Geometry check sheet. Reference: the model listing, model coordinates, mm. A direction names the side the tool comes from. Coordinates: 2 decimals unless noted, no trailing zeros. Order: outer loops, then holes, each group sorted by start corner. A loop starts at its lowest first (then second) coordinate and runs counter-clockwise, first axis right, second up. Notation, with made-up numbers: (18, 31) -> (65, 31) arc R17 cw to (65, 59) -> close; hole circle Ø5 at (-26, 2.5). An arc over 180 degrees is marked (long way). Answer in a Markdown table with one row per item. Add a question column.
```python
from build123d import *

# Parameters (mm, degrees)
ESQUISSE1_W        = 200
ESQUISSE1_H        = 200
BOSS_EXTRU_1_DEPTH = 50
ESQUISSE2_R        = 29
BOSS_EXTRU_2_DEPTH = 100


with BuildPart() as part:
    # Esquisse1 → Boss.-Extru.1 (new body)
    with BuildSketch(Plane.XY):
        Rectangle(ESQUISSE1_W, ESQUISSE1_H)
    extrude(amount=BOSS_EXTRU_1_DEPTH)

    # Esquisse2 → Boss.-Extru.2 (add)
    with BuildSketch(Plane.XY.offset(50)):
        Circle(ESQUISSE2_R)
    extrude(amount=BOSS_EXTRU_2_DEPTH)


solid = part.part
```
(1) Scan lines: line 1 along Z through (x, y) = (22.5, -25.5); line 2 along Y through (x, z) = (-1, 120.5); line 3 along X through (y, z) = (1.5, 133). Record each from-to range of solid material in increasing order.
(2) Cross-section at A-A (x = 0). Enter the section's corners in (y, z).
(3) Go/stop test with flat-tipped pins: P1, Ø10, axis at x = 4, z = 74.5, coming from the +Y side; P2, Ø1, axis at x = 14.5, y = -46.5, coming from the +Z side. Record where each tip stops, or that it passes through.
(4) Cross-section at C-C (z = 55). Enter the section's corners in (x, y), plus the area to 3 significant figures.
(5) Cross-section at D-D (y = -42.5). Enter the section's corners in (x, z), plus the area to 3 significant figures.
(6) Access from +Z, -Z, +X, -X, +Y, -Y to the whole of each face (thin tool, end or side, straight path). Record for faces 1 (the face through (13.38, -25.73, 99.3)), 2 (the face through (-1, 100, 25)).
Checks:
| question | item | result |
|---|---|---|
| 1 | line 1 | 0 to 50 |
| 1 | line 2 | -28.98 to 28.98 |
| 1 | line 3 | -28.96 to 28.96 |
| 2 | outline | (-100, 0) -> (100, 0) -> (100, 50) -> (29, 50) -> (29, 150) -> (-29, 150) -> (-29, 50) -> (-100, 50) -> close |
| 3 | P1 | y = 29 |
| 3 | P2 | z = 50 |
| 4 | outline | circle Ø58 at (0, 0) |
| 4 | area | 2,640 mm² |
| 5 | outline | (-100, 0) -> (100, 0) -> (100, 50) -> (-100, 50) -> close |
| 5 | area | 10,000 mm² |
| 6 | face 1 | +Z |
| 6 | face 2 | +Z, -Z, +X, -X, +Y |
